```python
from build123d import *

# Parameters (mm, degrees)
SKETCH2_R          = 0.9
CUT_EXTRUDE1_DEPTH = 31.347981811
CIRPATTERN1_COUNT  = 3


with BuildPart() as part:
    # Sketch1 → Revolve1 (revolve)
    with BuildSketch(Plane(origin=(0, 0, 0), x_dir=(1, 0, 0), z_dir=(0, 1, 0)), mode=Mode.PRIVATE) as revolve1_sk:
        Polygon((0, 5), (27, 5), (27, 14), (23, 14), (23, 9.5), (5, 9.5), (5, 8), (0, 8), align=None)
    revolve(revolve1_sk.sketch.rotate(Axis((0, 0, 0), (1, 0, 0)), 180), axis=Axis((0, 0, 0), (1, 0, 0)))

    # Sketch2 → Cut-Extrude1 (cut, through all)
    with BuildSketch(Plane.ZY.offset(-23)):
        with Locations((-11.75, 0)):
            Circle(SKETCH2_R)
    cut_extrude1 = extrude(amount=-CUT_EXTRUDE1_DEPTH, mode=Mode.SUBTRACT)

    # CirPattern1: Cut-Extrude1 ×3 about axis
    cirpattern1_axis = Axis((0, 0, 0), (1, 0, 0))
    for i in range(1, CIRPATTERN1_COUNT):
        add(cut_extrude1.rotate(cirpattern1_axis, i * 360 / CIRPATTERN1_COUNT), mode=Mode.SUBTRACT)


solid = part.part
```
CAD build for the part. Positions are in the model's coordinates, mm. A direction names the side the tool comes from. Coordinates: 2 decimals unless noted, no trailing zeros. Order: outer loops, then holes, each group sorted by start corner. A loop starts at its lowest first (then second) coordinate and runs counter-clockwise, first axis right, second up. Notation, with made-up numbers: M -27,-37 L 14,-37 A14 ccw 14,-21 Z; hole C -31.5,75 d6. An arc over 180 degrees is marked long. Answer as CSV lines item,"result".
1) Flat gauge pins, fed straight in: P1, Ø1.6, axis at y = 0, z = -11.75, coming from the +X side; P2, Ø4, axis at x = 8.5, y = 8, coming from the -Z side; P3, Ø1, axis at x = 24, y = -2.5, coming from the +Z side; P4, Ø3, axis at y = -10, z = 8.5, coming from the -X side. Where does each tip first touch, or does it go through?
Verdict:
P1,"through"
P2,"z = -7.37"
P3,"z = 13.86"
P4,"x = 23"
2) Cut at C-C (x = 21.25). List the corners of the cut face in (y, z).
Verdict:
outline,"C 0,0 d19; hole C 0,0 d10"
3) Drill centre lines: L1, parallel to Z at x = 23.25, y = -0.75; L2, parallel to X at y = 3.25, z = -7.75; L3, parallel to X at y = -4.5, z = 8.5. Where is each one in solid material? Low to high. Write a range as from..to.
Verdict:
L1,"-13.98..-12.25, -11.25..-4.94, 4.94..13.98"
L2,"5..27"
L3,"23..27"
4) Mould opens along Y. For faces 1 (the cylindrical face through (14, 0, -5)), 2 (the flat face through (27, 6, 0)), 3 (the cylindrical face through (24.972, 5.362, 12.932)) say: released by +Y, released by -Y, zero draft, split by the parting line, or undercut.
Verdict:
face 1,"undercut"
face 2,"zero draft"
face 3,"split by the parting line"
5) Cut at A-A (y = 0). List the corners of the cut face in (x, z), then the cut area to 3 significant figures.
Verdict:
outline,"M 0,-8 L 5,-8 L 5,-9.5 L 23,-9.5 L 23,-10.85 L 27,-10.85 L 27,-5 L 0,-5 Z; M 0,5 L 27,5 L 27,14 L 23,14 L 23,9.5 L 5,9.5 L 5,8 L 0,8 Z; M 23,-14 L 27,-14 L 27,-12.65 L 23,-12.65 Z"
area,"257 mm2"
6) Cut at D-D (z = -3). List the corners of the cut face in (x, y), then the cut area to 3 significant figures.
Verdict:
outline,"M 0,-7.42 L 5,-7.42 L 5,-9.01 L 23,-9.01 L 23,-13.67 L 27,-13.67 L 27,-4 L 0,-4 Z; M 0,4 L 27,4 L 27,13.67 L 23,13.67 L 23,9.01 L 5,9.01 L 5,7.42 L 0,7.42 Z"
area,"292 mm2"
7) Cut at B-B (y = -3.75). List the corners of the cut face in (x, z).
Verdict:
outline,"M 0,-7.07 L 5,-7.07 L 5,-8.73 L 23,-8.73 L 23,-13.49 L 27,-13.49 L 27,-3.31 L 0,-3.31 Z; M 0,3.31 L 27,3.31 L 27,13.49 L 23,13.49 L 23,8.73 L 5,8.73 L 5,7.07 L 0,7.07 Z"
8) 3-axis set-ups, long thin cutter, end or side, ignore diameter. For faces 4 (the cylindrical face through (2.46, 7.81, -1.73)), 5 (the cylindrical face through (24.972, 10.935, 6.359)): which of +Z, -Z, +X, -X, +Y, -Y reach the whole face in a straight line?
Verdict:
face 4,"-X"
face 5,"+X, -X"
